```python
from build123d import *

# Parameters (mm, degrees)
SKETCH1_W           = 558.8
SKETCH1_H           = 736.6
BOSS_EXTRUDE1_DEPTH = 50
SCALE1_SCALE        = 0.04


with BuildPart() as part:
    # Sketch1 → Boss-Extrude1 (new body)
    with BuildSketch(Plane.XY):
        Polygon((4705.35, 2489.2), (5226.05, 2489.2), (5226.05, 2540), (5746.75, 2540), (5746.75, 2489.2), (6267.45, 2489.2), (6267.45, 2540), (6788.15, 2540), (6788.15, 2489.2), (7308.85, 2489.2), (7308.85, 2540), (7829.55, 2540), (7829.55, 2489.2), (8350.25, 2489.2), (8350.25, 2540), (8890, 2540), (8890, 2051.05), (8839.2, 2051.05), (8839.2, 1530.35), (8890, 1530.35), (8890, 1009.65), (8839.2, 1009.65), (8839.2, 488.95), (8890, 488.95), (8890, 0), (8350.25, 0), (8350.25, 50.8), (7829.55, 50.8), (7829.55, 0), (7308.85, 0), (7308.85, 50.8), (6788.15, 50.8), (6788.15, 0), (6267.45, 0), (6267.45, 50.8), (5746.75, 50.8), (5746.75, 0), (5226.05, 0), (5226.05, 50.8), (4705.35, 50.8), (4705.35, 0), (4184.65, 0), (4184.65, 50.8), (3663.95, 50.8), (3663.95, 0), (3143.25, 0), (3143.25, 50.8), (2622.55, 50.8), (2622.55, 0), (2101.85, 0), (2101.85, 50.8), (1581.15, 50.8), (1581.15, 0), (1060.45, 0), (1060.45, 50.8), (539.75, 50.8), (539.75, 0), (0, 0), (0, 488.95), (50.8, 488.95), (50.8, 1009.65), (0, 1009.65), (0, 1530.35), (50.8, 1530.35), (50.8, 2051.05), (0, 2051.05), (0, 2540), (539.75, 2540), (539.75, 2489.2), (1060.45, 2489.2), (1060.45, 2540), (1581.15, 2540), (1581.15, 2489.2), (2101.85, 2489.2), (2101.85, 2540), (2622.55, 2540), (2622.55, 2489.2), (3143.25, 2489.2), (3143.25, 2540), (3663.95, 2540), (3663.95, 2489.2), (4184.65, 2489.2), (4184.65, 2540), (4705.35, 2540), align=None)
        Polygon((4470.4, 1231.9), (4419.6, 1231.9), (4415.704496234, 1232.096705982), (4411.921521072, 1232.674056618), (4404.769760674, 1234.894086722), (4398.297927796, 1238.406881576), (4392.659231682, 1243.059231682), (4388.006881576, 1248.697927542), (4384.494086976, 1255.16976042), (4382.274056618, 1262.321521072), (4381.696705982, 1266.104496234), (4381.5, 1270), (4381.696705982, 1273.895503512), (4382.274056618, 1277.678478928), (4384.494086976, 1284.830239326), (4388.006881576, 1291.302072204), (4392.659231682, 1296.940768318), (4398.297927796, 1301.593118424), (4404.769760674, 1305.105913024), (4411.921521072, 1307.325943382), (4415.704496234, 1307.903294018), (4419.6, 1308.1), (4470.4, 1308.1), (4474.295503766, 1307.903294018), (4478.078478928, 1307.325943382), (4485.230239326, 1305.105913024), (4491.702072204, 1301.593118424), (4497.340768318, 1296.940768318), (4501.993118424, 1291.302072204), (4505.505913024, 1284.830239326), (4507.725943382, 1277.678478928), (4508.303294018, 1273.895503512), (4508.5, 1270), (4508.303294018, 1266.104496234), (4507.725943382, 1262.321521072), (4505.505913024, 1255.16976042), (4501.993118424, 1248.697927542), (4497.340768318, 1243.059231682), (4491.702072204, 1238.406881576), (4485.230239326, 1234.894086722), (4478.078478928, 1232.674056618), (4474.295503766, 1232.096705982), align=None, mode=Mode.SUBTRACT)
        with Locations((7885.605536606, 1270)):
            Rectangle(SKETCH1_W, SKETCH1_H, mode=Mode.SUBTRACT)
    extrude(amount=BOSS_EXTRUDE1_DEPTH)


with BuildPart() as part_1:
    # Scale1: scaled about (4379.531045071, 1270, 25)
    add(part.part.scale(SCALE1_SCALE).moved(Location((4204.349803268, 1219.2, 24))))


solid = part_1.part
```
The model under review builds one solid part; all positions refer to its coordinate system, in mm. Round coordinates to 2 decimals unless told otherwise and drop trailing zeros. Loops run counter-clockwise (first coordinate to the right, second up) from the corner with the lowest first, then second, coordinate; pieces in that order, holes last. Notation, with made-up numbers: (-13, -26.75) -> (24, -26.75) arc R23 ccw to (24, -11.75) -> close; hole circle Ø3 at (4.25, 32.25). An arc over 180 degrees is marked (long way). Answer in a Markdown table with one row per item.
1) Consider section B-B, the plane z = 24.3. Count the separate pieces of the cut face and the enclosed holes in it, plus the area to 3 significant figures.
Taken from the geometry:
| item | result |
|---|---|
| separate pieces | 1 |
| enclosed holes | 2 |
| area | 34,600 mm² |
2) For pin 1 Ø1 at (x, z) = (4276.5, 24.5) entering from -Y; pin 2 Ø0.6 at (x, z) = (4484.5, 25) entering from +Y; pin 3 Ø1 at (y, z) = (1246.5, 25) entering from +X, all flat-tipped, find the tip position at first contact; note any pin that passes through.
Taken from the geometry:
| item | result |
|---|---|
| pin 1 | stops at y = 1221.23 |
| pin 2 | stops at y = 1318.77 |
| pin 3 | stops at x = 4557.92 |
3) Wall thickness on line 1 along X through (y, z) = (1273.5, 25.1); line 2 along X through (y, z) = (1280.5, 24.6); line 3 along Y through (x, z) = (4236, 25.8): over which ranges is each line inside the solid? List them lowest first.
Taken from the geometry:
| item | result |
|---|---|
| line 1 | x = 4204.35 to 4508.6, 4530.95 to 4559.95 |
| line 2 | x = 4206.38 to 4508.6, 4530.95 to 4557.92 |
| line 3 | y = 1221.23 to 1318.77 |
4) Consider section A-A, the plane y = 1263. Write out the cut boundary in (x, z).
Taken from the geometry:
| item | result |
|---|---|
| outline | (4204.35, 24) -> (4508.6, 24) -> (4508.6, 26) -> (4204.35, 26) -> close; (4530.95, 24) -> (4559.95, 24) -> (4559.95, 26) -> (4530.95, 26) -> close |
5) Consider section C-C, the plane x = 4359. Write out the cut boundary in (y, z).
Taken from the geometry:
| item | result |
|---|---|
| outline | (1221.23, 24) -> (1318.77, 24) -> (1318.77, 26) -> (1221.23, 26) -> close |
